Check sheet for the drawn part. Datum: minimum x, y, z corner. Units: mm. A direction names the side the tool comes from. Round coordinates to 2 decimals unless told otherwise and drop trailing zeros. Write each loop counter-clockwise with the first axis right and the second up, starting at its lowest first coordinate (ties: lowest second). Pieces come first, ordered by that corner, then holes. Notation, with made-up numbers: M 26.5,4 L 73.5,4 A16 cw 73.5,14 Z; hole C 75,-1 d1. An arc over 180 degrees is marked long. One line per item, written item: value. Start each with the question number.
Item 1: Draft check along X on the marked faces 3, 4 and 5. Enter one of: +X half, -X half, draft (parallel to the pull), parting line (faces both ways), or undercut.
Item 2: Thickness scan on probe 1 along Y at (x, z) = (12.5, 2.15); probe 2 along Z at (x, y) = (7.75, 6); probe 3 along Y at (x, z) = (4.5, 1.35) (1 decimal). Record the ranges inside material, lowest first. Write a range as from..to.
Item 3: Section check D-D, the plane x = 5. Record the cut outline in (y, z), then the cut area to 3 significant figures.
Item 4: Section check A-A, the plane y = 12.5. Record the cut outline in (x, z), then the cut area to 3 significant figures.
Item 5: Tool access check on the marked faces 1 and 2. Record the directions out of +Z, -Z, +X, -X, +Y, -Y that give a thin tool (end or side, any length) a straight path to the whole face; none if there is none.
Item 6: Gauge pin test, flat ends, axial feed: pin 1 (3.5 mm diameter, centred on x = 12.5, y = 4.5, fed in from +Z); pin 2 (1.5 mm diameter, centred on y = 14.5, z = 6, fed in from -X); pin 3 (5 mm diameter, centred on x = 15, z = 4, fed in from +Y). Record the tip position at first contact, or that the pin passes through.
Item 7: Section check C-C, the plane z = 5. Record the cut outline in (x, y), then the cut area to 3 significant figures.
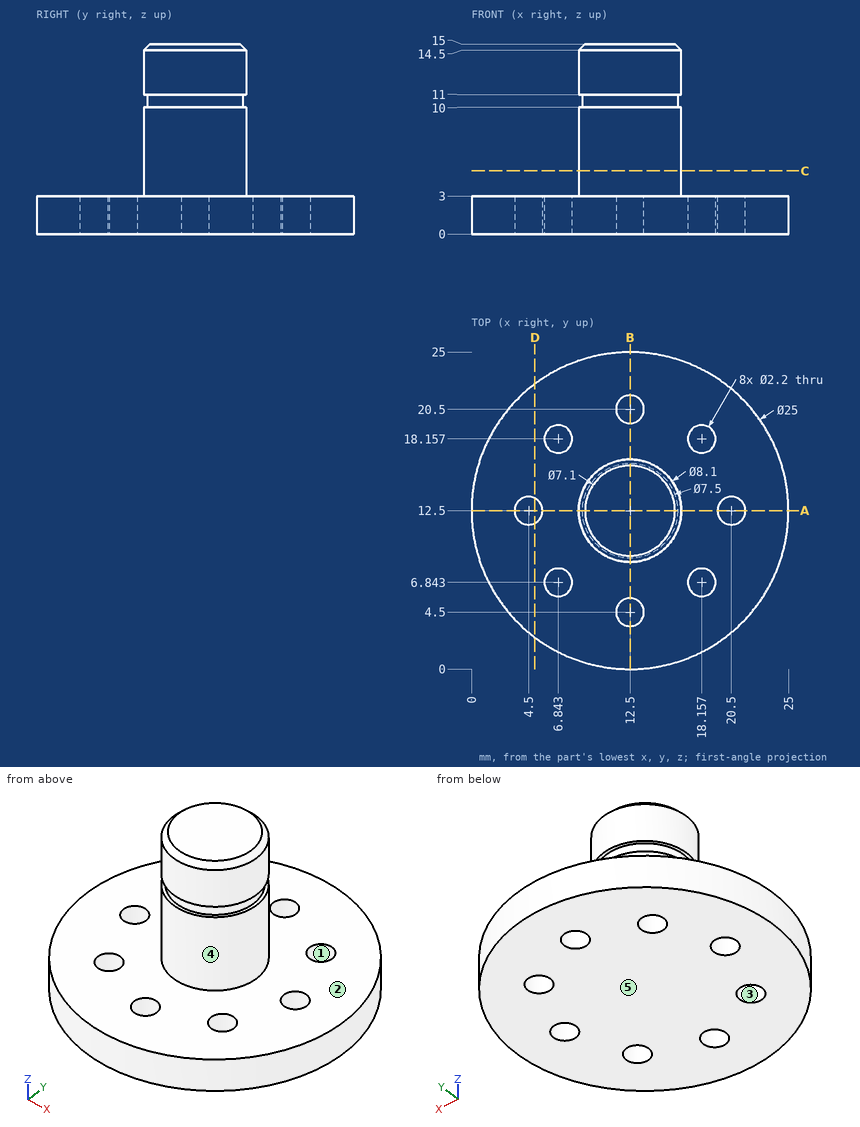
Response values:
1. face 3: undercut
1. face 4: parting line
1. face 5: draft
2. probe 1: y = 0..3.4, 5.6..19.4, 21.6..25
2. probe 2: z = 0..3
2. probe 3: y = 2.9..11.4, 13.6..22.1
3. outline: M 2.5,0 L 11.52,0 L 11.52,3 L 2.5,3 Z; M 13.48,0 L 22.5,0 L 22.5,3 L 13.48,3 Z
3. area: 54.1 mm2
4. outline: M 0,0 L 3.4,0 L 3.4,3 L 0,3 Z; M 5.6,0 L 19.4,0 L 19.4,3 L 16.55,3 L 16.55,10 L 16.25,10 L 16.25,11 L 16.55,11 L 16.55,14.5 L 16.05,15 L 8.95,15 L 8.45,14.5 L 8.45,11 L 8.75,11 L 8.75,10 L 8.45,10 L 8.45,3 L 5.6,3 Z; M 21.6,0 L 25,0 L 25,3 L 21.6,3 Z
4. area: 158 mm2
5. face 1: +Z, -Z
5. face 2: +Z
6. pin 1: stops at z = 3
6. pin 2: stops at x = 8.65
6. pin 3: stops at y = 25
7. outline: C 12.5,12.5 d8.1
7. area: 51.5 mm2
